from build123d import *

# Parameters (mm, degrees)
SKETCH1_W           = 25
SKETCH1_H           = 40
BOSS_EXTRUDE1_DEPTH = 50
SKETCH2_W           = 22.5
SKETCH2_H           = 40
CUT_EXTRUDE1_DEPTH  = 25
SKETCH3_W           = 20
SKETCH3_H           = 10
CUT_EXTRUDE2_DEPTH  = 10
SKETCH5_R           = 1
CUT_EXTRUDE4_DEPTH  = 12
SKETCH6_W           = 25
SKETCH6_H           = 40
CUT_EXTRUDE5_DEPTH  = 8
SKETCH7_W           = 20
SKETCH7_H           = 22.5
CUT_EXTRUDE6_DEPTH  = 8
SKETCH8_R           = 1.8
CUT_EXTRUDE7_DEPTH  = 8
SKETCH12_W          = 10
SKETCH12_H          = 10
CUT_EXTRUDE9_DEPTH  = 10
SKETCH13_W          = 2.5
SKETCH13_H          = 40
BOSS_EXTRUDE2_DEPTH = 19
SKETCH14_W          = 40
SKETCH14_H          = 61
BOSS_EXTRUDE3_DEPTH = 2
SKETCH15_W          = 40
SKETCH15_H          = 3
BOSS_EXTRUDE4_DEPTH = 22.5
SKETCH16_W          = 10
SKETCH16_H          = 3
CUT_EXTRUDE10_DEPTH = 22.5
SKETCH17_W          = 10
SKETCH17_H          = 54
CUT_EXTRUDE11_DEPTH = 5.5
SKETCH18_W          = 27
SKETCH18_H          = 30
BOSS_EXTRUDE5_DEPTH = 10
SKETCH19_W          = 30
SKETCH19_H          = 71
BOSS_EXTRUDE6_DEPTH = 5
SKETCH20_W          = 32
SKETCH20_H          = 10
CUT_EXTRUDE12_DEPTH = 13


with BuildPart() as part:
    # Sketch1 → Boss-Extrude1 (new body)
    with BuildSketch(Plane(origin=(0, 0, 0), x_dir=(1, 0, 0), z_dir=(0, 1, 0))):
        with Locations((12.5, 20)):
            Rectangle(SKETCH1_W, SKETCH1_H)
    extrude(amount=BOSS_EXTRUDE1_DEPTH)

    # Sketch2 → Cut-Extrude1 (cut)
    with BuildSketch(Plane(origin=(0, 50, 0), x_dir=(1, 0, 0), z_dir=(0, 1, 0))):
        with Locations((13.75, 20)):
            Rectangle(SKETCH2_W, SKETCH2_H)
    extrude(amount=-CUT_EXTRUDE1_DEPTH, mode=Mode.SUBTRACT)

    # Sketch3 → Cut-Extrude2 (cut)
    with BuildSketch(Plane.XY):
        with Locations((12.5, 20)):
            Rectangle(SKETCH3_W, SKETCH3_H)
    extrude(amount=-CUT_EXTRUDE2_DEPTH, mode=Mode.SUBTRACT)

    # Sketch5 → Cut-Extrude4 (cut)
    with BuildSketch(Plane.XY.offset(-10)):
        with Locations((7.5, 21)):
            Circle(SKETCH5_R)
        with Locations((17.5, 21)):
            Circle(SKETCH5_R)
    cut_extrude4 = extrude(amount=-CUT_EXTRUDE4_DEPTH, mode=Mode.SUBTRACT)

    # Sketch6 → Cut-Extrude5 (cut)
    with BuildSketch(Plane.XZ):
        with Locations((12.5, -20)):
            Rectangle(SKETCH6_W, SKETCH6_H)
    extrude(amount=-CUT_EXTRUDE5_DEPTH, mode=Mode.SUBTRACT)

    # Sketch7 → Cut-Extrude6 (cut)
    with BuildSketch(Plane.XZ.offset(-8)):
        with Locations((12.5, -26.25)):
            Rectangle(SKETCH7_W, SKETCH7_H)
    extrude(amount=-CUT_EXTRUDE6_DEPTH, mode=Mode.SUBTRACT)

    # Sketch8 → Cut-Extrude7 (cut, through all)
    with BuildSketch(Plane(origin=(0, 15, 0), x_dir=(1, 0, 0), z_dir=(0, 1, 0))):
        with Locations((7.5, 3.5)):
            Circle(SKETCH8_R)
        with Locations((17.5, 3.5)):
            Circle(SKETCH8_R)
    extrude(amount=-CUT_EXTRUDE7_DEPTH, mode=Mode.SUBTRACT)

    # Sketch12 → Cut-Extrude9 (cut)
    with BuildSketch(Plane.ZY.offset(-22.5)):
        with Locations((-5, 20)):
            Rectangle(SKETCH12_W, SKETCH12_H)
    extrude(amount=-CUT_EXTRUDE9_DEPTH, mode=Mode.SUBTRACT)

    # Sketch13 → Boss-Extrude2 (add)
    with BuildSketch(Plane(origin=(0, 50, 0), x_dir=(1, 0, 0), z_dir=(0, 1, 0))):
        with Locations((1.25, 20)):
            Rectangle(SKETCH13_W, SKETCH13_H)
    extrude(amount=BOSS_EXTRUDE2_DEPTH)

    # Sketch14 → Boss-Extrude3 (add)
    with BuildSketch(Plane.ZY):
        with Locations((-20, 38.5)):
            Rectangle(SKETCH14_W, SKETCH14_H)
    extrude(amount=BOSS_EXTRUDE3_DEPTH)

    # Sketch15 → Boss-Extrude4 (add)
    with BuildSketch(Plane(origin=(2.5, 0, 0), x_dir=(0, 0, -1), z_dir=(1, 0, 0))):
        with Locations((20, 67.5)):
            Rectangle(SKETCH15_W, SKETCH15_H)
    extrude(amount=BOSS_EXTRUDE4_DEPTH)

    # Sketch16 → Cut-Extrude10 (cut)
    with BuildSketch(Plane(origin=(25, 0, 0), x_dir=(0, 0, -1), z_dir=(1, 0, 0))):
        with Locations((5, 67.5)):
            Rectangle(SKETCH16_W, SKETCH16_H)
    extrude(amount=-CUT_EXTRUDE10_DEPTH, mode=Mode.SUBTRACT)

    # Sketch17 → Cut-Extrude11 (cut, through all)
    with BuildSketch(Plane(origin=(2.5, 0, 0), x_dir=(0, 0, -1), z_dir=(1, 0, 0))):
        with Locations((5, 42)):
            Rectangle(SKETCH17_W, SKETCH17_H)
    extrude(amount=-CUT_EXTRUDE11_DEPTH, mode=Mode.SUBTRACT)

    # Sketch18 → Boss-Extrude5 (add)
    with BuildSketch(Plane(origin=(0, 69, 0), x_dir=(1, 0, 0), z_dir=(0, 1, 0))):
        with Locations((11.5, 25)):
            Rectangle(SKETCH18_W, SKETCH18_H)
    extrude(amount=BOSS_EXTRUDE5_DEPTH)

    # Mirror1: Cut-Extrude4 across plane
    add(cut_extrude4.mirror(Plane(origin=(0, 45.25, 0), x_dir=(0, 0, 1), z_dir=(0, -1, 0))), mode=Mode.SUBTRACT)

    # Sketch19 → Boss-Extrude6 (add)
    with BuildSketch(Plane.ZY.offset(2)):
        with Locations((-25, 43.5)):
            Rectangle(SKETCH19_W, SKETCH19_H)
    extrude(amount=BOSS_EXTRUDE6_DEPTH)

    # Sketch20 → Cut-Extrude12 (cut)
    with BuildSketch(Plane(origin=(0, 79, 0), x_dir=(1, 0, 0), z_dir=(0, 1, 0))):
        with Locations((9, 35)):
            Rectangle(SKETCH20_W, SKETCH20_H)
    extrude(amount=-CUT_EXTRUDE12_DEPTH, mode=Mode.SUBTRACT)


solid = part.part
Input: part model. Units: mm. Frame: model coordinates. A direction names the side the tool comes from. Coordinates: 2 decimals unless noted, no trailing zeros. Loops run counter-clockwise (first coordinate to the right, second up) from the corner with the lowest first, then second, coordinate; pieces in that order, holes last.
Q1. Contact query for flat-ended pins moving along their axis: pin 1 (5 mm diameter, centred on x = 10, y = 25, fed in from +Z); pin 2 (4.5 mm diameter, centred on x = 7.5, z = -3.5, fed in from -Y); pin 3 (1.6 mm diameter, centred on x = 17.5, y = 21, fed in from +Z); pin 4 (4 mm diameter, centred on x = 16, y = 72.5, fed in from -Z). Output: stop coordinate, or through.
Q2. Material intervals for line 1 (Y direction, x = 7.5, z = -15.75); line 2 (Y direction, x = 7.5, z = -14.75); line 3 (Z direction, x = 7.5, y = 13.25), sorted ascending.
Q3. Draft query along Y for faces 6 (the face through (14, 25, -25)), 7 (the face through (17.266, 11.549, -5.285)), 8 (the face through (9, 79, -20)), 9 (the face through (17, 69, -22)). Return one class per face: +Y half, -Y half, draft (parallel to the pull), parting line (faces both ways), or undercut.
Q4. Set-up query: faces 1 (the face through (2.5, 12, -26)), 2 (the face through (25, 72, -20)), 3 (the face through (-7, 44, -25)), 4 (the face through (7.96, 70.39, -15.92)), 5 (the face through (-2, 66, -35)). Return all of +Z, -Z, +X, -X, +Y, -Y with unobstructed straight access to the full face (end or side cutting, diameter ignored); none if empty.
Q5. Cut plane D-D (y = 21). Output: boundary loops of the cut face in (x, z), then the cut area to 3 significant figures.
Q6. Cut plane A-A (z = -18). Output: boundary loops of the cut face in (x, y), then the cut area to 3 significant figures.
Q7. Cut plane B-B (x = 7.5). Output: boundary loops of the cut face in (y, z), then the cut area to 3 significant figures.
Q8. Cut plane C-C (z = -3.5). Output: boundary loops of the cut face in (x, y), then the cut area to 3 significant figures.
Working result:
1. pin 1: stops at z = -10
1. pin 2: stops at y = 8
1. pin 3: stops at z = -22
1. pin 4: stops at z = -30
2. line 1: y = 16 to 20, 22 to 25, 66 to 68.5, 70.5 to 79
2. line 2: y = 8 to 20, 22 to 25, 66 to 68.5, 70.5 to 79
2. line 3: z = -40 to -37.5, -15 to -5.3, -1.7 to 0
3. face 6: undercut
3. face 7: draft
3. face 8: +Y half
3. face 9: undercut
4. face 1: -Y
4. face 2: +Z, -Z, +X, +Y, -Y
4. face 3: +Z, -Z, -X, +Y, -Y
4. face 4: +Z
4. face 5: -Z, +X, -X, +Y
5. outline: (-7, -40) - (25, -40) - (25, -10) - (18.5, -10) - (18.5, -22) - (16.5, -22) - (16.5, -10) - (8.5, -10) - (8.5, -22) - (6.5, -22) - (6.5, -10) - (-7, -10) - close
5. area: 912 mm2
6. outline: (-7, 8) - (2.5, 8) - (2.5, 16) - (22.5, 16) - (22.5, 8) - (25, 8) - (25, 25) - (2.5, 25) - (2.5, 66) - (25, 66) - (25, 79) - (-7, 79) - close; hole circle Ø2 at (7.5, 21); hole circle Ø2 at (7.5, 69.5); hole circle Ø2 at (17.5, 21); hole circle Ø2 at (17.5, 69.5)
6. area: 1,180 mm2
7. outline: (8, -40) - (25, -40) - (25, -10) - (22, -10) - (22, -22) - (20, -22) - (20, -10) - (15, -10) - (15, -5.3) - (8, -5.3) - (8, -15) - (16, -15) - (16, -37.5) - (8, -37.5) - close; (8, -1.7) - (15, -1.7) - (15, 0) - (8, 0) - close; (66, -30) - (79, -30) - (79, -10) - (70.5, -10) - (70.5, -22) - (68.5, -22) - (68.5, -10) - (66, -10) - close
7. area: 587 mm2
8. outline: (-2, 8) - (5.7, 8) - (5.7, 15) - (-2, 15) - close; (9.3, 8) - (15.7, 8) - (15.7, 15) - (9.3, 15) - close; (19.3, 8) - (25, 8) - (25, 15) - (19.3, 15) - close
8. area: 139 mm2
